```python
from build123d import *

# Parameters (mm, degrees)
SKETCH1_R           = 16
SKETCH1_R_2         = 1.6
BOSS_EXTRUDE1_DEPTH = 43


with BuildPart() as part:
    # Sketch1 → Boss-Extrude1 (new body)
    with BuildSketch(Plane.XY):
        Circle(SKETCH1_R)
        with Locations((-8, -8)):
            Circle(SKETCH1_R_2, mode=Mode.SUBTRACT)
        with Locations((8, -8)):
            Circle(SKETCH1_R_2, mode=Mode.SUBTRACT)
        with Locations((-8, 8)):
            Circle(SKETCH1_R_2, mode=Mode.SUBTRACT)
        with BuildLine():
            Line((-3.605551275, -6), (-6, -6))
            Line((-6, -6), (-6, -3.605551275))
            ThreePointArc((-6, -3.605551275), (-7, 0), (-6, 3.605551275))
            Line((-6, 3.605551275), (-6, 6))
            Line((-6, 6), (-3.605551275, 6))
            ThreePointArc((-3.605551275, 6), (0, 7), (3.605551275, 6))
            Line((3.605551275, 6), (6, 6))
            Line((6, 6), (6, 3.605551275))
            ThreePointArc((6, 3.605551275), (6.745368782, 1.870828693), (7, 0))
            ThreePointArc((7, 0), (6.745368782, -1.870828693), (6, -3.605551275))
            Line((6, -3.605551275), (6, -6))
            Line((6, -6), (3.605551275, -6))
            ThreePointArc((3.605551275, -6), (0, -7), (-3.605551275, -6))
        make_face(mode=Mode.SUBTRACT)
        with Locations((8, 8)):
            Circle(SKETCH1_R_2, mode=Mode.SUBTRACT)
    extrude(amount=BOSS_EXTRUDE1_DEPTH)


solid = part.part
```
The model under review builds one solid part; all positions refer to its coordinate system, in mm. A direction names the side the tool comes from. Coordinates: 2 decimals unless noted, no trailing zeros. Order: outer loops, then holes, each group sorted by start corner. A loop starts at its lowest first (then second) coordinate and runs counter-clockwise, first axis right, second up. Notation, with made-up numbers: (87.5, 60.5) -> (113.5, 60.5) arc R27 cw to (113.5, 76.5) -> close; hole circle Ø1 at (71, -23). An arc over 180 degrees is marked (long way). Answer in a Markdown table with one row per item. Add a question column.
Item 1: Clearance check with flat-ended pins moving along their axes: pin 1 (1.9 mm diameter, centred on x = -4.5, z = 30, fed in from -Y); pin 2 (1.9 mm diameter, centred on y = 5, z = 20, fed in from +X); pin 3 (2 mm diameter, centred on y = -10.5, z = 38.5, fed in from -X). State where each tip first meets the part, or that it passes through.
Item 2: Machinability: for faces 1 (the flat face through (6, -5, 21)), 2 (the flat face through (7, -3, 0)), which of the approach directions +Z, -Z, +X, -X, +Y, -Y give a long, thin tool a straight path to every point of the face, cutting with its end or side? Answer none if there is none.
Item 3: To check wall thickness, follow probe 1 along Y at (x, z) = (-8, 11); probe 2 along X at (y, z) = (9, 32); probe 3 along Y at (x, z) = (2, 32). State the ranges of each line that lie inside material, in increasing order.
Item 4: Mouldability with a two-part tool opening along Y and no side actions: class faces 3 (the cylindrical face through (0, 7, 21)), 4 (the flat face through (7, -3, 43)), 5 (the cylindrical face through (-3.47, -15.62, 21.2)) as +Y half, -Y half, draft (parallel to the pull), parting line (faces both ways), or undercut.
Item 5: We need section B-B on y = -8. Write out the cut boundary in (x, z), plus the area to 3 significant figures.
Item 6: We need section A-A on z = 18.5. Write out the cut boundary in (x, y), plus the area to 3 significant figures.
Item 7: We need section C-C on x = 4.5. Write out the cut boundary in (y, z), plus the area to 3 significant figures.
Final values:
| question | item | result |
|---|---|---|
| 1 | pin 1 | stops at y = -15.6 |
| 1 | pin 2 | stops at x = 15.48 |
| 1 | pin 3 | stops at x = -12.87 |
| 2 | face 1 | +Z, -Z |
| 2 | face 2 | -Z, +X, -X, +Y, -Y |
| 3 | probe 1 | y = -13.86 to -9.6, -6.4 to 6.4, 9.6 to 13.86 |
| 3 | probe 2 | x = -13.23 to -9.25, -6.75 to 6.75, 9.25 to 13.23 |
| 3 | probe 3 | y = -15.87 to -6.71, 6.71 to 15.87 |
| 4 | face 3 | undercut |
| 4 | face 4 | draft |
| 4 | face 5 | parting line |
| 5 | outline | (-13.86, 0) -> (-9.6, 0) -> (-9.6, 43) -> (-13.86, 43) -> close; (-6.4, 0) -> (6.4, 0) -> (6.4, 43) -> (-6.4, 43) -> close; (9.6, 0) -> (13.86, 0) -> (13.86, 43) -> (9.6, 43) -> close |
| 5 | area | 916 mm2 |
| 6 | outline | circle Ø32 at (0, 0); hole circle Ø3.2 at (-8, -8); hole circle Ø3.2 at (-8, 8); hole (-6, -6) -> (-3.61, -6) arc R7 ccw to (3.61, -6) -> (6, -6) -> (6, -3.61) arc R7 ccw to (6, 3.61) -> (6, 6) -> (3.61, 6) arc R7 ccw to (-3.61, 6) -> (-6, 6) -> (-6, 3.61) arc R7 ccw to (-6, -3.61) -> close; hole circle Ø3.2 at (8, -8); hole circle Ø3.2 at (8, 8) |
| 6 | area | 609 mm2 |
| 7 | outline | (-15.35, 0) -> (-6, 0) -> (-6, 43) -> (-15.35, 43) -> close; (6, 0) -> (15.35, 0) -> (15.35, 43) -> (6, 43) -> close |
| 7 | area | 804 mm2 |
